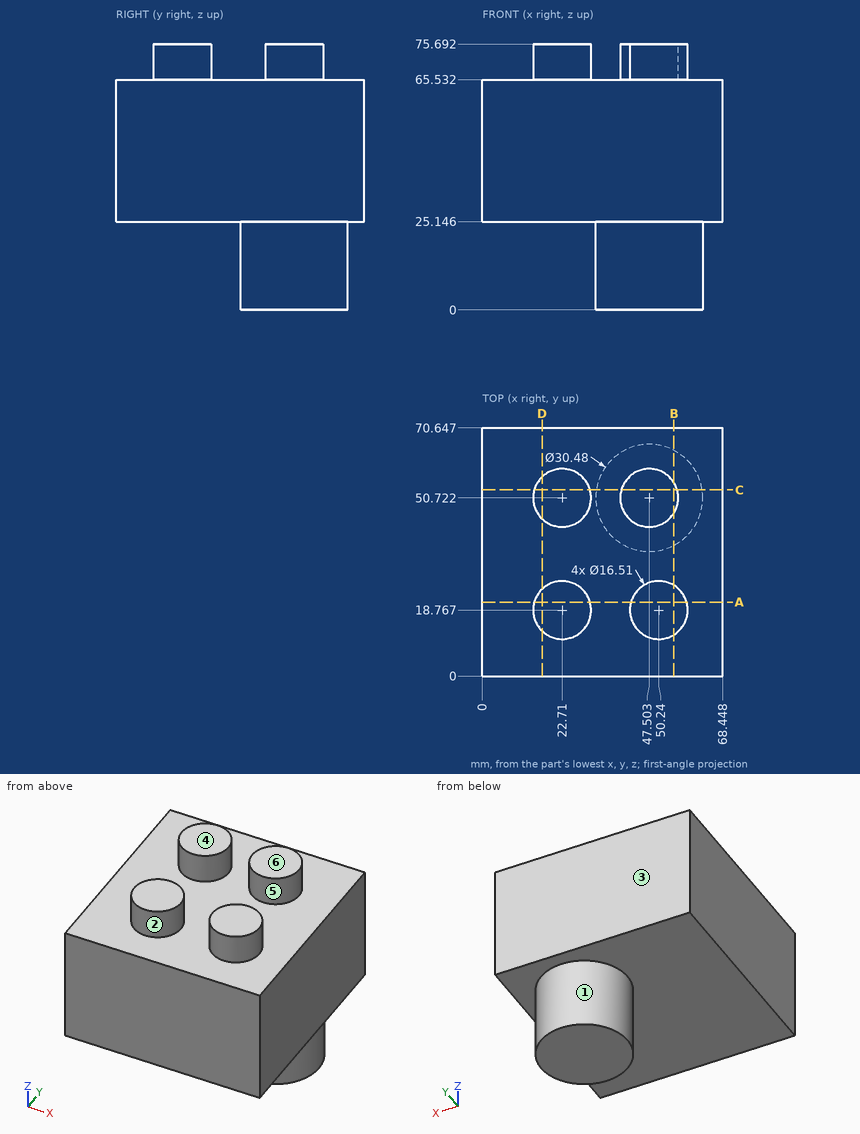
Here's the drawing with two shaded views (mm, measured from the low corner). I have some questions. A direction names the side the tool comes from. Coordinates: 2 decimals unless noted, no trailing zeros. Write each loop counter-clockwise with the first axis right and the second up, starting at its lowest first coordinate (ties: lowest second). Pieces come first, ordered by that corner, then holes. Notation, with made-up numbers: (76.5, 68.5) -> (114.5, 68.5) arc R11 cw to (114.5, 89.5) -> close; hole circle Ø2 at (5.25, 9). An arc over 180 degrees is marked (long way). Write item = value, one per line. Start each with the question number.
(1) I want a section at C-C (y = 53). Please give me the cut outline in (x, z) (1 decimal), plus the area to 3 significant figures.
(2) Which directions (+Z, -Z, +X, -X, +Y, -Y) give clear straight access to the entire face, cutting with the end or side of a thin tool? Please do the marked faces 5 and 6.
(3) I want a section at D-D (x = 17). Please give me the cut outline in (y, z) (1 decimal).
(4) I want a section at A-A (y = 21). Please give me the cut outline in (x, z) (1 decimal).
(5) We'd pull the mould along Y, two halves only. Please class the marked faces 1, 2, 3 and 4: released by +Y, released by -Y, zero draft, split by the parting line, or undercut.
(6) Will these pins go through, and if not, where does the flat tip stop? pin 1 (3 mm diameter, centred on x = 21.5, y = 18.5, fed in from -Z); pin 2 (8 mm diameter, centred on x = 40.5, z = 15, fed in from +Y); pin 3 (10 mm diameter, centred on x = 9.5, y = 56.5, fed in from +Z).
(7) I want a section at B-B (x = 54.5). Please give me the cut outline in (y, z) (1 decimal), plus the area to 3 significant figures.
(8) I need wall thicknesses on line 1 (Z direction, x = 25, y = 46) (1 decimal); line 2 (Z direction, x = 29, y = 63) (1 decimal); line 3 (Y direction, x = 50, z = 68) (1 decimal). Which ranges of each line are inside material? Lowest first, please. Write a range as [from, to].
Result set:
q1.outline = (0, 25.1) -> (32.4, 25.1) -> (32.4, 0) -> (62.6, 0) -> (62.6, 25.1) -> (68.4, 25.1) -> (68.4, 65.5) -> (55.4, 65.5) -> (55.4, 75.7) -> (39.6, 75.7) -> (39.6, 65.5) -> (30.6, 65.5) -> (30.6, 75.7) -> (14.8, 75.7) -> (14.8, 65.5) -> (0, 65.5) -> close
q1.area = 3,840 mm2
q2.face_5 = +Z
q2.face_6 = +Z, +X, -X, +Y, -Y
q3.outline = (0, 25.1) -> (70.6, 25.1) -> (70.6, 65.5) -> (56.7, 65.5) -> (56.7, 75.7) -> (44.8, 75.7) -> (44.8, 65.5) -> (24.7, 65.5) -> (24.7, 75.7) -> (12.8, 75.7) -> (12.8, 65.5) -> (0, 65.5) -> close
q4.outline = (0, 25.1) -> (68.4, 25.1) -> (68.4, 65.5) -> (58.2, 65.5) -> (58.2, 75.7) -> (42.3, 75.7) -> (42.3, 65.5) -> (30.7, 65.5) -> (30.7, 75.7) -> (14.8, 75.7) -> (14.8, 65.5) -> (0, 65.5) -> close
q5.face_1 = split by the parting line
q5.face_2 = undercut
q5.face_3 = released by +Y
q5.face_4 = zero draft
q6.pin_1 = 25.15
q6.pin_2 = 65.66
q6.pin_3 = 65.53
q7.outline = (0, 25.1) -> (37.2, 25.1) -> (37.2, 0) -> (64.3, 0) -> (64.3, 25.1) -> (70.6, 25.1) -> (70.6, 65.5) -> (55.1, 65.5) -> (55.1, 75.7) -> (46.3, 75.7) -> (46.3, 65.5) -> (25.8, 65.5) -> (25.8, 75.7) -> (11.7, 75.7) -> (11.7, 65.5) -> (0, 65.5) -> close
q7.area = 3,770 mm2
q8.line_1 = [25.1, 75.7]
q8.line_2 = [25.1, 65.5]
q8.line_3 = [10.5, 27], [42.9, 58.6]
